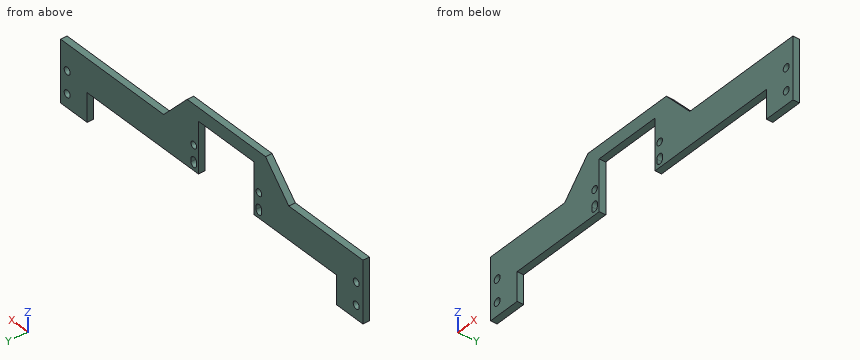
```python
from build123d import *

# Parameters (mm, degrees)
SKETCH_1_R      = 2.25
SKETCH_1_R_2    = 2.1
EXTRUDE_1_DEPTH = 4
EXTRUDE_2_DEPTH = 4


with BuildPart() as part:
    # 草图1 → 凸台-拉伸1 (new body)
    with BuildSketch(Plane(origin=(0, 0, 0), x_dir=(1, 0, 0), z_dir=(0, 1, 0))):
        Polygon((-83.136892884, -5.45556523), (-125.136892884, -5.45556523), (-125.136892884, 25.54443477), (-186.886892884, 25.54443477), (-186.886892884, 43.04443477), (-206.886892884, 43.04443477), (-206.886892884, 5.54443477), (-189.553457543, 5.54443477), (-133.636892884, 5.54443477), (-133.636892884, -13.45556523), (-74.636892884, -13.45556523), (-74.636892884, 5.54443477), (1.279671775, 5.54443477), (20.613107116, 5.54443477), (20.613107116, 13.09443477), (20.613107116, 43.04443477), (0.613107116, 43.04443477), (0.613107116, 25.54443477), (-74.636892884, 25.54443477), (-83.136892884, 25.54443477), align=None)
        with Locations((15.613107116, 34.84443477)):
            Circle(SKETCH_1_R, mode=Mode.SUBTRACT)
        with Locations((15.613107116, 21.34443477)):
            Circle(SKETCH_1_R, mode=Mode.SUBTRACT)
        with Locations((-79.636892884, 10.54443477)):
            Circle(SKETCH_1_R_2, mode=Mode.SUBTRACT)
        with Locations((-128.636892884, 10.54443477)):
            Circle(SKETCH_1_R_2, mode=Mode.SUBTRACT)
        with Locations((-201.886892884, 34.84443477)):
            Circle(SKETCH_1_R, mode=Mode.SUBTRACT)
        with Locations((-201.886892884, 21.34443477)):
            Circle(SKETCH_1_R, mode=Mode.SUBTRACT)
        with BuildLine():
            Line((-81.736892884, 21.54443477), (-81.736892884, 19.54443477))
            ThreePointArc((-81.736892884, 19.54443477), (-79.636892884, 17.44443477), (-77.536892884, 19.54443477))
            Line((-77.536892884, 19.54443477), (-77.536892884, 21.54443477))
            ThreePointArc((-77.536892884, 21.54443477), (-79.636892884, 23.64443477), (-81.736892884, 21.54443477))
        make_face(mode=Mode.SUBTRACT)
        with BuildLine():
            Line((-130.736892884, 21.54443477), (-130.736892884, 19.54443477))
            ThreePointArc((-130.736892884, 19.54443477), (-128.636892884, 17.44443477), (-126.536892884, 19.54443477))
            Line((-126.536892884, 19.54443477), (-126.536892884, 21.54443477))
            ThreePointArc((-126.536892884, 21.54443477), (-128.636892884, 23.64443477), (-130.736892884, 21.54443477))
        make_face(mode=Mode.SUBTRACT)
    extrude(amount=EXTRUDE_1_DEPTH)

    # 草图4 → 凸台-拉伸2 (add)
    with BuildSketch(Plane(origin=(0, 4, 0), x_dir=(1, 0, 0), z_dir=(0, 1, 0))):
        Polygon((-133.636892884, -13.45556523), (-151.115738533, 5.54443477), (-133.636892884, 5.54443477), align=None)
        Polygon((-74.636892884, -13.45556523), (-74.636892884, 5.54443477), (-56.979755625, 5.54443477), align=None)
    extrude(amount=-EXTRUDE_2_DEPTH)


solid = part.part
```
Could you check a few things on this model? Use its own coordinates, in mm. Coordinates: 2 decimals unless noted, no trailing zeros. Loops run counter-clockwise (first coordinate to the right, second up) from the corner with the lowest first, then second, coordinate; pieces in that order, holes last. Notation, with made-up numbers: M 61.25,80 L 114.25,80 A24 ccw 114.25,104 Z; hole C -15,65 d10. An arc over 180 degrees is marked long. Put each result on its own line as item: value. Start each with the question number.
(1) Will these pins go through, and if not, where does the flat tip stop? P1, Ø1.5, axis at y = 1, z = -4, coming from the +X side; P2, Ø1, axis at x = -148, y = 2.5, coming from the -Z side; P3, Ø2, axis at x = -98.5, y = 3.5, coming from the -Z side; P4, Ø4, axis at x = -79.64, z = -10.54, coming from the +Y side.
(2) Suppose I cut it at C-C on x = -106. Please give me the cut outline in (y, z).
(3) Suppose I cut it at B-B on y = 2.35. Count the separate pieces of the cut face and the enclosed holes in it, then the cut area to 3 significant figures.
(4) I need wall thicknesses on line 1 (Z direction, x = -79.5, y = 0.95); line 2 (X direction, y = 0.75, z = -25); line 3 (X direction, y = 1.7, z = -22.5). Which ranges of each line are inside material? Lowest first, please. Write a range as from..to.
(5) Suppose I cut it at A-A on z = -30. Please give me the cut outline in (x, y), then the cut area to 3 significant figures.
(6) Suppose I cut it at D-D on x = 2.5. Please give me the cut outline in (y, z).
Solutions:
1. P1: stops at x = -57.72
1. P2: stops at z = -25.54
1. P3: stops at z = 5.46
1. P4: passes through
2. outline: M 0,5.46 L 4,5.46 L 4,13.46 L 0,13.46 Z
3. separate pieces: 1
3. enclosed holes: 8
3. area: 5,270 mm2
4. line 1: z = -25.54..-23.64, -17.45..-12.64, -8.45..13.46
4. line 2: x = -206.89..-125.14, -83.14..20.61
4. line 3: x = -206.89..-203.82, -199.96..-130.51, -126.77..-125.14, -83.14..-81.51, -77.77..13.68, 17.54..20.61
5. outline: M -206.89,0 L -186.89,0 L -186.89,4 L -206.89,4 Z; M 0.61,0 L 20.61,0 L 20.61,4 L 0.61,4 Z
5. area: 160 mm2
6. outline: M 0,-43.04 L 4,-43.04 L 4,-5.54 L 0,-5.54 Z
